from build123d import *

# Parameters (mm, degrees)
F0_W        = 110
F0_H        = 25
F1_DEPTH    = 5.55
F2_R        = 2
F3_DEPTH    = 2
F4_R        = 1.5
F5_DEPTH    = 1
F6_DEPTH    = 2
F8_T1_DEPTH = 139.9155060128
F8_T3_DEPTH = 54.9155060128


# Not quite as in the source:
# - a fillet or chamfer that OpenCascade refuses, or shapes differently, is made with other operations: its cross-section is extruded or revolved along the edge and cut away or added


with BuildPart() as f1:
    # F0 (on Front) → F1 (new body)
    with BuildSketch(Plane.XZ):
        Rectangle(F0_W, F0_H)
    extrude(amount=F1_DEPTH)

    # F2 (on face) → F3 (cut)
    with BuildSketch(Plane.XZ.offset(5.55)):
        with Locations((-49, 0)):
            Circle(F2_R)
    extrude(amount=-F3_DEPTH, mode=Mode.SUBTRACT)

    # F4 (on face) → F5 (join)
    with BuildSketch(Plane.XZ.offset(5.55)):
        with Locations((0, 9.82276164)):
            Circle(F4_R)
        with Locations((-51.5013597906, 9.6743786708)):
            Circle(F4_R)
        with Locations((47.8420853615, 9.8438328132)):
            Circle(F4_R)
    extrude(amount=F5_DEPTH)

    # F4 (on face) → F6 (join)
    with BuildSketch(Plane.XZ.offset(5.55)):
        with Locations((0, 9.82276164)):
            Circle(F4_R)
        with Locations((-51.5013597906, 9.6743786708)):
            Circle(F4_R)
        with Locations((47.8420853615, 9.8438328132)):
            Circle(F4_R)
    extrude(amount=F6_DEPTH)

    # F7: F1 across face


with BuildPart() as f1_1:
    add(f1.part)
    add(f1.part.mirror(Plane(origin=(0, -7.55, 9.82276164), x_dir=(1, 0, 0), z_dir=(0, -1, 0))))

    # F8: fillet of radius 6 on 8 edges, made by hand

    # F8_s2 → F8_t1 (cut)
    with BuildSketch(Plane.YZ.offset(-69.9577530064)):
        with BuildLine():
            ThreePointArc((-9.55, -12.5), (-13.4988634896, -10.5973399501), (-15.1, -6.5168987974))
            Line((-15.1, -6.5168987974), (-15.1, -12.5))
            Line((-15.1, -12.5), (-9.55, -12.5))
        make_face()
        with BuildLine():
            ThreePointArc((-9.55, 12.5), (-13.4988634896, 10.5973399501), (-15.1, 6.5168987974))
            Line((-15.1, 6.5168987974), (-15.1, 12.5))
            Line((-15.1, 12.5), (-9.55, 12.5))
        make_face()
        with BuildLine():
            ThreePointArc((-5.55, -12.5), (-1.6011365104, -10.5973399501), (0, -6.5168987974))
            Line((0, -6.5168987974), (0, -12.5))
            Line((0, -12.5), (-5.55, -12.5))
        make_face()
        with BuildLine():
            ThreePointArc((0, 6.5168987974), (-1.6011365104, 10.5973399501), (-5.55, 12.5))
            Line((-5.55, 12.5), (0, 12.5))
            Line((0, 12.5), (0, 6.5168987974))
        make_face()
    extrude(amount=F8_T1_DEPTH, mode=Mode.SUBTRACT)

    # F8_s4 → F8_t3 (cut)
    with BuildSketch(Plane.XY.offset(-27.4577530064)):
        with BuildLine():
            ThreePointArc((55, -9.55), (53.0973399501, -13.4988634896), (49.0168987974, -15.1))
            Line((49.0168987974, -15.1), (55, -15.1))
            Line((55, -15.1), (55, -9.55))
        make_face()
        with BuildLine():
            ThreePointArc((-55, -9.55), (-53.0973399501, -13.4988634896), (-49.0168987974, -15.1))
            Line((-49.0168987974, -15.1), (-55, -15.1))
            Line((-55, -15.1), (-55, -9.55))
        make_face()
        with BuildLine():
            ThreePointArc((55, -5.55), (53.0973399501, -1.6011365104), (49.0168987974, 0))
            Line((49.0168987974, 0), (55, 0))
            Line((55, 0), (55, -5.55))
        make_face()
        with BuildLine():
            ThreePointArc((-55, -5.55), (-53.0973399501, -1.6011365104), (-49.0168987974, 0))
            Line((-49.0168987974, 0), (-55, 0))
            Line((-55, 0), (-55, -5.55))
        make_face()
    extrude(amount=F8_T3_DEPTH, mode=Mode.SUBTRACT)


solid = f1_1.part
Here's how the part is built. I have some questions about the finished solid (model axes, mm). A direction names the side the tool comes from. Give positions to 0.01 mm unless a question says otherwise; leave off trailing zeros. Order: outer loops, then holes, each group sorted by start corner. A loop starts at its lowest first (then second) coordinate and runs counter-clockwise, first axis right, second up. Notation, with made-up numbers: M 30,-34 L 46,-34 A21 ccw 46,2 Z; hole C -17,31.5 d8. An arc over 180 degrees is marked long. Answer as a JSON object with one key per item and string values. Group by question number.
1) I'm going to push a flat-ended pin straight in: pin 1 Ø1.5 at (y, z) = (-12.5, -6.5) entering from +X. Where does the tip first touch, or does it pass through?
2) Suppose I cut it at A-A, the plane z = 0. Write out the boundary of the cut face in (x, y), plus the area to 3 significant figures.
3) Suppose I cut it at B-B, the plane x = -45. Write out the boundary of the cut face in (y, z), plus the area to 3 significant figures.
4) We'd pull the mould along X, two halves only. Please class faces 3 (the cylindrical face through (-0.77, -13.46, 10.64)), 4 (the flat face through (-49, -11.55, 0)), 5 (the cylindrical face through (-53.81, -2.39, -0.18)): pulls with the +X half, pulls with the -X half, needs draft (parallel to the pull), parting line crosses it, or undercut.
5) Suppose I cut it at C-C, the plane x = 0. Write out the boundary of the cut face in (y, z).
6) Please list where these lines run through material, in increasing order: L1, parallel to Y at x = 2.5, z = 2.5; L2, parallel to Z at x = -49, y = -10.1; L3, parallel to Y at x = 8, z = 8.5. Write a range as [from, to].
7) On a 3-axis mill with a long thin cutter (end or side, diameter ignored), from which of +Z, -Z, +X, -X, +Y, -Y can I reach the whole of each face in a straight line? I mean faces 1 (the cylindrical face through (53.81, -12.71, -0.18)), 2 (the flat face through (-49, -3.55, 0)). Say none if no direction works.
8) Suppose I cut it at D-D, the plane y = -8.25. Write out the boundary of the cut face in (x, z).
Results found:
{
 "1": {"pin 1": "x = 54.4"},
 "2": {"outline": "M -55,-9.55 A6 ccw -49.02,-15.1 L 49.02,-15.1 A6 ccw 55,-9.55 L -47,-9.55 L -47,-11.55 L -51,-11.55 L -51,-9.55 Z; M -55,-5.55 L -51,-5.55 L -51,-3.55 L -47,-3.55 L -47,-5.55 L 55,-5.55 A6 ccw 49.02,0 L -49.02,0 A6 ccw Z", "area": "1,170 mm²"},
 "3": {"outline": "M -15.1,-6.52 A6 ccw -9.55,-12.5 L -9.55,12.5 A6 ccw -15.1,6.52 Z; M -5.55,-12.5 A6 ccw 0,-6.52 L 0,6.52 A6 ccw -5.55,12.5 Z", "area": "247 mm²"},
 "4": {"face 3": "needs draft", "face 4": "undercut", "face 5": "pulls with the -X half"},
 "5": {"outline": "M -15.1,-6.52 A6 ccw -9.55,-12.5 L -9.55,8.32 L -5.55,8.32 L -5.55,-12.5 A6 ccw 0,-6.52 L 0,6.52 A6 ccw -5.55,12.5 L -5.55,11.32 L -9.55,11.32 L -9.55,12.5 A6 ccw -15.1,6.52 Z"},
 "6": {"L1": "[-15.1, -9.55], [-5.55, 0]", "L2": "[-12.43, -2], [2, 12.43]", "L3": "[-14.76, -9.55], [-5.55, -0.34]"},
 "7": {"face 1": "+Z, -Z, +X, -Y", "face 2": "none"},
 "8": {"outline": "C -51.5,9.67 d3; C 0,9.82 d3; C 47.84,9.84 d3"}
}
